```python
from build123d import *

# Parameters (mm, degrees)
ESQUISSE1_W        = 37.5
ESQUISSE1_H        = 37.5
BOSS_EXTRU_1_DEPTH = 22.3
CONG_1_R           = 3
ESQUISSE2_R        = 17.5
BOSS_EXTRU_2_DEPTH = 13
ESQUISSE3_R        = 1.4
BOSS_EXTRU_3_DEPTH = 3.7


with BuildPart() as part:
    # Esquisse1 → Boss.-Extru.1 (new body)
    with BuildSketch(Plane(origin=(0, 0, 0), x_dir=(1, 0, 0), z_dir=(0, 1, 0))):
        Rectangle(ESQUISSE1_W, ESQUISSE1_H)
    extrude(amount=BOSS_EXTRU_1_DEPTH)

    # Congé1
    cong_1_edges = [part.edges().sort_by_distance(p)[0] for p in [
        (18.75, 11.15, 18.75),
        (-18.75, 11.15, 18.75),
        (-18.75, 11.15, -18.75),
        (18.75, 11.15, -18.75),
    ]]
    fillet(cong_1_edges, radius=CONG_1_R)

    # Esquisse2 → Boss.-Extru.2 (add)
    with BuildSketch(Plane(origin=(0, 22.3, 0), x_dir=(1, 0, 0), z_dir=(0, 1, 0))):
        Circle(ESQUISSE2_R)
    extrude(amount=BOSS_EXTRU_2_DEPTH)

    # Esquisse3 → Boss.-Extru.3 (add)
    with BuildSketch(Plane.XZ):
        with BuildLine():
            Line((-18.75, 14.5), (-23, 14.5))
            ThreePointArc((-23, 14.5), (-26.5, 11), (-23, 7.5))
            Line((-23, 7.5), (-18.75, 7.5))
            Line((-18.75, 7.5), (-18.75, 14.5))
        make_face()
        with Locations((-23, 11)):
            Circle(ESQUISSE3_R, mode=Mode.SUBTRACT)
        with BuildLine():
            Line((18.75, 7.5), (23, 7.5))
            ThreePointArc((23, 7.5), (26.5, 11), (23, 14.5))
            Line((23, 14.5), (18.75, 14.5))
            Line((18.75, 14.5), (18.75, 7.5))
        make_face()
        with Locations((23, 11)):
            Circle(ESQUISSE3_R, mode=Mode.SUBTRACT)
        with BuildLine():
            ThreePointArc((-3.5, -21.726136344), (0, -25.226136344), (3.5, -21.726136344))
            Line((3.5, -21.726136344), (3.5, -18.75))
            Line((3.5, -18.75), (-3.5, -18.75))
            Line((-3.5, -18.75), (-3.5, -21.726136344))
        make_face()
        with Locations((0, -21.726136344)):
            Circle(ESQUISSE3_R, mode=Mode.SUBTRACT)
    extrude(amount=-BOSS_EXTRU_3_DEPTH)


solid = part.part
```
Here's how the part is built. I have some questions about the finished solid (model axes, mm). A direction names the side the tool comes from. Coordinates: 2 decimals unless noted, no trailing zeros. Order: outer loops, then holes, each group sorted by start corner. A loop starts at its lowest first (then second) coordinate and runs counter-clockwise, first axis right, second up. Notation, with made-up numbers: (84.25, 58.25) -> (99.25, 58.25) arc R23 cw to (99.25, 94.25) -> close; hole circle Ø9 at (62.5, 45.5). An arc over 180 degrees is marked (long way). Return JSON: item names as keys, results as strings.
1) If we section it at B-B on z = 11: List the corners of the cut face in (x, y) for me, plus the area to 3 significant figures.
Conclusion:
{"outline": "(-26.5, 0) -> (-24.4, 0) -> (-24.4, 3.7) -> (-26.5, 3.7) -> close; (-21.6, 0) -> (21.6, 0) -> (21.6, 3.7) -> (18.75, 3.7) -> (18.75, 22.3) -> (13.61, 22.3) -> (13.61, 35.3) -> (-13.61, 35.3) -> (-13.61, 22.3) -> (-18.75, 22.3) -> (-18.75, 3.7) -> (-21.6, 3.7) -> close; (24.4, 0) -> (26.5, 0) -> (26.5, 3.7) -> (24.4, 3.7) -> close", "area": "1,230 mm²"}
2) If we section it at A-A on x = 0: List the corners of the cut face in (y, z) for me, plus the area to 3 significant figures.
Conclusion:
{"outline": "(0, -25.23) -> (3.7, -25.23) -> (3.7, -23.13) -> (0, -23.13) -> close; (0, -20.33) -> (3.7, -20.33) -> (3.7, -18.75) -> (22.3, -18.75) -> (22.3, -17.5) -> (35.3, -17.5) -> (35.3, 17.5) -> (22.3, 17.5) -> (22.3, 18.75) -> (0, 18.75) -> close", "area": "1,300 mm²"}
3) On a 3-axis mill with a long thin cutter (end or side, diameter ignored), from which of +Z, -Z, +X, -X, +Y, -Y can I reach the whole of each face in a straight line? I mean faces 1 (the flat face through (2, 3.7, -22)), 2 (the flat face through (-21, 2, 7.5)), 3 (the flat face through (-21, 2, 14.5)), 4 (the flat face through (-6, 22.3, -17)). Say none if no direction works.
Conclusion:
{"face 1": "-Z, +X, -X, +Y", "face 2": "-Z, -X, +Y, -Y", "face 3": "+Z, -X, +Y, -Y", "face 4": "+Y"}
4) If we section it at D-D on z = 0: List the corners of the cut face in (x, y) for me, plus the area to 3 significant figures.
Conclusion:
{"outline": "(-18.75, 0) -> (18.75, 0) -> (18.75, 22.3) -> (17.5, 22.3) -> (17.5, 35.3) -> (-17.5, 35.3) -> (-17.5, 22.3) -> (-18.75, 22.3) -> close", "area": "1,290 mm²"}
5) If we section it at C-C on y = 10: List the corners of the cut face in (x, z) for me, plus the area to 3 significant figures.
Conclusion:
{"outline": "(-18.75, -15.75) arc R3 ccw to (-15.75, -18.75) -> (15.75, -18.75) arc R3 ccw to (18.75, -15.75) -> (18.75, 15.75) arc R3 ccw to (15.75, 18.75) -> (-15.75, 18.75) arc R3 ccw to (-18.75, 15.75) -> close", "area": "1,400 mm²"}
6) Thinking about a two-plate mould opening in Z: for faces 5 (the cylindrical face through (-17.89, 11.31, 17.85)), 6 (the cylindrical face through (0.646, 1.824, -22.968)), 7 (the flat face through (21, 2, 7.5)), which applies, +Z half, -Z half, draft (parallel to the pull), parting line (faces both ways), or undercut?
Conclusion:
{"face 5": "+Z half", "face 6": "undercut", "face 7": "-Z half"}
7) I'm going to push flat-ended pins straight in: P1, Ø18, axis at x = -4, y = 13, coming from the -Z side; P2, Ø1.8, axis at x = -21.5, y = 2.5, coming from the +Z side; P3, Ø7, axis at x = 1.5, z = -21, coming from the +Y side; P4, Ø2.5, axis at x = 0, z = -21.73, coming from the +Y side. Where does each tip first touch, or does it pass through?
Conclusion:
{"P1": "stops at z = -18.75", "P2": "stops at z = 14.5", "P3": "stops at y = 22.3", "P4": "passes through"}
8) If I drill on probe 1 along Z at (x, y) = (23, 1); probe 2 along Z at (x, y) = (0, 2); probe 3 along Z at (x, y) = (-6.5, 10), over which ranges is the centre line in solid material (lowest first)?
Conclusion:
{"probe 1": "z = 7.5 to 9.6, 12.4 to 14.5", "probe 2": "z = -25.23 to -23.13, -20.33 to 18.75", "probe 3": "z = -18.75 to 18.75"}
